Read the model definition and answer for the solid it produces. Units are mm, in the model's axes. Face numbers are marked on the shaded views. Coordinates: 2 decimals unless noted, no trailing zeros. Write each loop counter-clockwise with the first axis right and the second up, starting at its lowest first coordinate (ties: lowest second). Pieces come first, ordered by that corner, then holes. Notation, with made-up numbers: (-4, -9) -> (34, -9) arc R16 ccw to (34, 1) -> close; hole circle Ø6 at (14, 28.25). An arc over 180 degrees is marked (long way). Answer as a JSON object with one key per item and string values. Group by question number.
(1) For a pull along Y with two mould halves and no side action, classify the marked faces 1, 2 and 3 as +Y half, -Y half, draft (parallel to the pull), parting line (faces both ways), or undercut.
(2) Find section A-A (z = -12.25). Give the vertices of the cut face in (x, y), then the cut area to 3 significant figures.
(3) Straight lines are drawn through the part: L1, parallel to Y at x = 0, z = -20; L2, parallel to Y at x = 19, z = -8.25; L3, parallel to X at y = 18, z = -2. For each, find the intervals that lie inside material, in ascending order.
(4) Flat-ended cylindrical pins translate along their axes: P1, Ø3, axis at x = 28, z = -12, coming from the -Y side; P2, Ø8, axis at y = 11, z = -7.5, coming from the -X side; P3, Ø4, axis at x = 10, y = 8, coming from the -Z side; P4, Ø3, axis at x = 47, z = -12.5, coming from the -Y side. Find the tip coordinate at first contact, or state that the pin passes through.
(5) Find section D-D (x = -0.66). Give the vertices of the cut face in (y, z), then the cut area to 3 significant figures.
(6) Find section C-C (z = -2). Give the vertices of the cut face in (x, y), then the cut area to 3 significant figures.
(7) Find section B-B (y = 10). Give the vertices of the cut face in (x, z), then the cut area to 3 significant figures.
from build123d import *

# Parameters (mm, degrees)
SKETCH1_R               = 4
BOSS_EXTRUDE1_DEPTH     = 25
FILLET1_R               = 5
SKETCH2_W               = 5
SKETCH2_H               = 30
CUT_EXTRUDE1_DEPTH      = 1.812260823
CUT_EXTRUDE1_DEPTH_BACK = 71.77899263


with BuildPart() as part:
    # Sketch1 → Boss-Extrude1 (new body)
    with BuildSketch(Plane.XY):
        with BuildLine():
            ThreePointArc((56.45524489, 48.144548452), (61.045451548, 58.48524489), (50.70475511, 63.075451548))
            Line((50.70475511, 63.075451548), (-3.53524489, 42.185451548))
            ThreePointArc((-3.53524489, 42.185451548), (-7.298349786, 39.184561806), (-8.658548629, 34.567619439))
            Line((-8.658548629, 34.567619439), (-8, 0))
            ThreePointArc((-8, 0), (0.076026565, -7.999638739), (7.99855499, 0.152046264))
            Line((7.99855499, 0.152046264), (7.445069005, 29.268763528))
            Line((7.445069005, 29.268763528), (56.45524489, 48.144548452))
        make_face()
        Circle(SKETCH1_R, mode=Mode.SUBTRACT)
        with Locations((-0.66, 34.72)):
            Circle(SKETCH1_R, mode=Mode.SUBTRACT)
        with Locations((53.58, 55.61)):
            Circle(SKETCH1_R, mode=Mode.SUBTRACT)
    extrude(amount=-BOSS_EXTRUDE1_DEPTH)

    # Fillet1
    fillet1_edges = [part.edges().sort_by_distance(p)[0] for p in [
        (7.445069005, 29.268763528, -12.5),
    ]]
    fillet(fillet1_edges, radius=FILLET1_R)

    # Sketch2 → Cut-Extrude1 (cut, two sides)
    with BuildSketch(Plane(origin=(-7.997097521, -0.152352916, 0), x_dir=(0, 0, 1), z_dir=(-0.999818579, -0.01904757, 0))) as cut_extrude1_sk:
        with Locations((-12.5, 2)):
            Rectangle(SKETCH2_W, SKETCH2_H)
    extrude(amount=CUT_EXTRUDE1_DEPTH, mode=Mode.SUBTRACT)
    extrude(cut_extrude1_sk.sketch, amount=-CUT_EXTRUDE1_DEPTH_BACK, mode=Mode.SUBTRACT)


solid = part.part
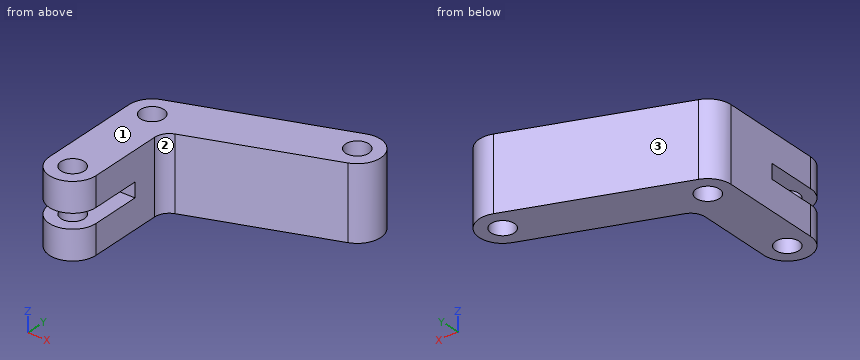
Results below:
{
 "1": {"face 1": "draft", "face 2": "undercut", "face 3": "+Y half"},
 "2": {"outline": "(-8.66, 34.57) -> (-8.32, 16.84) -> (7.68, 17.15) -> (7.51, 25.77) arc R5 cw to (10.71, 30.53) -> (56.46, 48.14) arc R8 ccw to (50.7, 63.08) -> (-3.54, 42.19) arc R8 ccw to start; hole circle Ø8 at (-0.66, 34.72); hole circle Ø8 at (53.58, 55.61)", "area": "1,210 mm2"},
 "3": {"L1": "y = -8 to -4, 4 to 30.77, 38.67 to 43.55", "L2": "y = 33.72 to 50.86", "L3": "x = -8.34 to 7.66"},
 "4": {"P1": "stops at y = 36.61", "P2": "stops at x = -8.29", "P3": "passes through", "P4": "stops at y = 43.93"},
 "5": {"outline": "(-7.97, -25) -> (-3.95, -25) -> (-3.95, -15) -> (-7.97, -15) -> close; (-7.97, -10) -> (-3.95, -10) -> (-3.95, 0) -> (-7.97, 0) -> close; (3.95, -25) -> (30.72, -25) -> (30.72, 0) -> (3.95, 0) -> (3.95, -10) -> (16.99, -10) -> (16.99, -15) -> (3.95, -15) -> close; (38.72, -25) -> (43.29, -25) -> (43.29, 0) -> (38.72, 0) -> close", "area": "799 mm2"},
 "6": {"outline": "(-8.66, 34.57) -> (-8, 0) arc R8 ccw (long way) to (8, 0.15) -> (7.51, 25.77) arc R5 cw to (10.71, 30.53) -> (56.46, 48.14) arc R8 ccw to (50.7, 63.08) -> (-3.54, 42.19) arc R8 ccw to start; hole circle Ø8 at (-0.66, 34.72); hole circle Ø8 at (0, 0); hole circle Ø8 at (53.58, 55.61)", "area": "1,530 mm2"},
 "7": {"outline": "(-8.19, -25) -> (7.81, -25) -> (7.81, -15) -> (-8.19, -15) -> close; (-8.19, -10) -> (7.81, -10) -> (7.81, 0) -> (-8.19, 0) -> close", "area": "320 mm2"}
}
